Part model, mm, in its own coordinate system. A direction names the side the tool comes from. Round coordinates to 2 decimals unless told otherwise and drop trailing zeros. Write each loop counter-clockwise with the first axis right and the second up, starting at its lowest first coordinate (ties: lowest second). Pieces come first, ordered by that corner, then holes.
```python
from build123d import *

# Parameters (mm, degrees)
BOSS_EXTRUDE1_DEPTH = 22.86
SKETCH3_R           = 27.372592865
CUT_EXTRUDE1_DEPTH  = 69.240761179
SKETCH4_R           = 26.837944266
CUT_EXTRUDE2_DEPTH  = 64.339651167
BOSS_EXTRUDE2_START = 22.86
SKETCH2_3_W         = 2.286
SKETCH2_3_H         = 2.286
SKETCH2_3_R         = 1.05
SKETCH2_3_H_2       = 9.395
BOSS_EXTRUDE2_DEPTH = 12.7
SKETCH5_W           = 49.53
SKETCH5_H           = 1.9
CUT_EXTRUDE4_DEPTH  = 46.736
SKETCH6_W           = 51.181
SKETCH6_H           = 10.146462019
CUT_EXTRUDE5_DEPTH  = 74.476087969


with BuildPart() as part:
    # Sketch2 → Boss-Extrude1 (new body)
    with BuildSketch(Plane(origin=(0, 0, 0), x_dir=(1, 0, 0), z_dir=(0, 1, 0))):
        Polygon((29.493, -25.5905), (29.493, 25.5905), (20.857, 25.5905), (20.857, -13.9095), (-20.857, -13.9095), (-20.857, 25.5905), (-29.493, 25.5905), (-29.493, -25.5905), align=None)
    extrude(amount=BOSS_EXTRUDE1_DEPTH)

    # Sketch3 → Cut-Extrude1 (cut, through all)
    with BuildSketch(Plane(origin=(29.493, 0, 0), x_dir=(0, 0, -1), z_dir=(1, 0, 0))):
        with Locations((2.032, -17.226130846)):
            Circle(SKETCH3_R)
        Polygon((25.5905, 12.7), (-21.1455, 12.7), (-21.1455, 18.796), (25.5905, 18.034), align=None)
    extrude(amount=-CUT_EXTRUDE1_DEPTH, mode=Mode.SUBTRACT)

    # Sketch4 → Cut-Extrude2 (cut, through all)
    with BuildSketch(Plane(origin=(0, 0, -25.5905), x_dir=(-1, 0, 0), z_dir=(0, 0, -1))):
        with Locations((0, -16.88966558)):
            Circle(SKETCH4_R)
    extrude(amount=-CUT_EXTRUDE2_DEPTH, mode=Mode.SUBTRACT)

    # Sketch2_3 → Boss-Extrude2 (add)
    with BuildSketch(Plane(origin=(0, 0, 0), x_dir=(1, 0, 0), z_dir=(0, 1, 0)).offset(BOSS_EXTRUDE2_START)):
        with Locations((22, 24.4475)):
            Rectangle(SKETCH2_3_W, SKETCH2_3_H)
        with Locations((22, 24.4475)):
            Circle(SKETCH2_3_R, mode=Mode.SUBTRACT)
        with Locations((22, -15.0525)):
            Rectangle(SKETCH2_3_W, SKETCH2_3_H)
        with Locations((22, -15.0525)):
            Circle(SKETCH2_3_R, mode=Mode.SUBTRACT)
        with Locations((-22, -15.0525)):
            Rectangle(SKETCH2_3_W, SKETCH2_3_H)
        with Locations((-22, -15.0525)):
            Circle(SKETCH2_3_R, mode=Mode.SUBTRACT)
        with Locations((-22, 24.4475)):
            Rectangle(SKETCH2_3_W, SKETCH2_3_H)
        with Locations((-22, 24.4475)):
            Circle(SKETCH2_3_R, mode=Mode.SUBTRACT)
        Polygon((29.493, 25.5905), (23.143, 25.5905), (23.143, 23.3045), (23.143, -13.9095), (23.143, -16.1955), (23.143, -25.5905), (29.493, -25.5905), align=None)
        with Locations((22, -20.893)):
            Rectangle(SKETCH2_3_W, SKETCH2_3_H_2)
        with Locations((-22, -20.893)):
            Rectangle(SKETCH2_3_W, SKETCH2_3_H_2)
        Polygon((-23.143, 23.3045), (-23.143, 25.5905), (-29.493, 25.5905), (-29.493, -25.5905), (-23.143, -25.5905), (-23.143, -16.1955), (-23.143, -13.9095), align=None)
        with Locations((22, -15.0525)):
            Circle(SKETCH2_3_R)
        with Locations((22, 24.4475)):
            Circle(SKETCH2_3_R)
        Polygon((23.143, -13.9095), (23.143, 23.3045), (20.857, 23.3045), (20.857, 4.6975), (20.857, -13.9095), align=None)
        Polygon((-20.857, 4.6975), (-20.857, 23.3045), (-23.143, 23.3045), (-23.143, -13.9095), (-20.857, -13.9095), align=None)
        with Locations((-22, 24.4475)):
            Circle(SKETCH2_3_R)
        with Locations((-22, -15.0525)):
            Circle(SKETCH2_3_R)
    extrude(amount=BOSS_EXTRUDE2_DEPTH)

    # Sketch5 → Cut-Extrude4 (cut)
    with BuildSketch(Plane(origin=(0, 0, -25.5905), x_dir=(-1, 0, 0), z_dir=(0, 0, -1))):
        with Locations((0, 32.61)):
            Rectangle(SKETCH5_W, SKETCH5_H)
    extrude(amount=-CUT_EXTRUDE4_DEPTH, mode=Mode.SUBTRACT)

    # Sketch6 → Cut-Extrude5 (cut, through all)
    with BuildSketch(Plane(origin=(29.493, 0, 0), x_dir=(0, 0, -1), z_dir=(1, 0, 0))):
        with Locations((0, 5.07323101)):
            Rectangle(SKETCH6_W, SKETCH6_H)
    extrude(amount=-CUT_EXTRUDE5_DEPTH, mode=Mode.SUBTRACT)


solid = part.part
```
Q1. Cut at B-B on x = 25.5. Write the cut outline in (y, z).
Values follow:
outline: (10.15, -25.59) - (12.7, -25.59) - (12.7, 21.15) - (18.8, 21.15) - (18.03, -25.59) - (35.56, -25.59) - (35.56, 25.59) - (10.15, 25.59) - close
Q2. Cut at D-D on y = 29. Write the cut outline in (x, z), plus the area to 3 significant figures.
Values follow:
outline: (-29.49, -25.59) - (-20.86, -25.59) - (-20.86, 25.59) - (-29.49, 25.59) - close; (20.86, -25.59) - (29.49, -25.59) - (29.49, 25.59) - (20.86, 25.59) - close
area: 884 mm2
Q3. Wall check: L1, parallel to X at y = 29, z = -22.5; L2, parallel to X at y = 31.75, z = -13 (3 decimals); L3, parallel to Z at x = -4.5, y = 11.25. Give the ranges that are in metal, low to high.
Values follow:
L1: x = -29.49 to -20.86, 20.86 to 29.49
L2: x = -29.493 to -24.765, 24.765 to 29.493
L3: z = 13.91 to 25.59
Q4. Cut at C-C on z = 13. Write the cut outline in (x, y) (3 decimals).
Values follow:
outline: (-29.493, 10.146) - (-20.857, 10.146) - (-20.857, 12.7) - (-29.493, 12.7) - close; (-29.493, 18.663) - (-20.857, 18.663) - (-20.857, 31.66) - (-24.765, 31.66) - (-24.765, 33.56) - (-20.857, 33.56) - (-20.857, 35.56) - (-29.493, 35.56) - close; (20.857, 10.146) - (29.493, 10.146) - (29.493, 12.7) - (20.857, 12.7) - close; (20.857, 18.663) - (29.493, 18.663) - (29.493, 35.56) - (20.857, 35.56) - (20.857, 33.56) - (24.765, 33.56) - (24.765, 31.66) - (20.857, 31.66) - close
Q5. Drop flat-ended pins along their axis: pin 1 (2 mm diameter, centred on x = -4, y = 11, fed in from -Z); pin 2 (9.5 mm diameter, centred on x = 0, z = 18.5, fed in from +Y). Give the stop position or say it passes through.
Values follow:
pin 1: stops at z = 13.91
pin 2: stops at y = 22.86
Q6. Cut at A-A on y = 32.5. Write the cut outline in (x, z) (1 decimal).
Values follow:
outline: (-29.5, -25.6) - (-24.8, -25.6) - (-24.8, 21.1) - (-20.9, 21.1) - (-20.9, 25.6) - (-29.5, 25.6) - close; (20.9, 21.1) - (24.8, 21.1) - (24.8, -25.6) - (29.5, -25.6) - (29.5, 25.6) - (20.9, 25.6) - close
Q7. Which spindle directions (+Z, -Z, +X, -X, +Y, -Y) get a long thin tool onto all of the face, cutting with end or side? Do faces 5 (the flat face through (-23, 31.66, -3)), 6 (the flat face through (20.857, 27, 0)), 7 (the flat face through (0, 22.86, 20)), 8 (the flat face through (20.857, 11, -6)). Say none if no direction does.
Values follow:
face 5: -Z
face 6: -Z, +Y
face 7: +Z, -Z, +Y
face 8: -Z, +Y, -Y
Q8. Mould opens along X. For faces 1 (the flat face through (-23, 33.56, -3)), 2 (the flat face through (29.493, 25, 0)), 3 (the flat face through (-23, 33, 21.146)), 4 (the flat face through (0, 20, 25.59)) say: +X half, -X half, draft (parallel to the pull), parting line (faces both ways), or undercut.
Values follow:
face 1: undercut
face 2: +X half
face 3: undercut
face 4: draft
